Build history of the part. All positions in model axes, mm. Face numbers are marked on the shaded views. A direction names the side the tool comes from. Coordinates: 2 decimals unless noted, no trailing zeros. Order: outer loops, then holes, each group sorted by start corner. A loop starts at its lowest first (then second) coordinate and runs counter-clockwise, first axis right, second up. Notation, with made-up numbers: (19.25, 21.25) -> (68.25, 21.25) arc R33 ccw to (68.25, 54.25) -> close; hole circle Ø10 at (24.25, 24). An arc over 180 degrees is marked (long way). Write each question's results on one line, items separated by ' | '.
from build123d import *

# Parameters (mm, degrees)
F0_W     = 25
F0_H     = 1
F0_W_2   = 76
F0_W_3   = 75
F3_R     = 55
F4_DEPTH = 176
F5_R     = 75
F6_DEPTH = 1200


# Not quite as in the source:
# - a feature names something its author has since deleted; it is built from what else it names


with BuildPart() as f1:
    # F0 (on Front) → F1 (revolve)
    with BuildSketch(Plane.XZ):
        Polygon((-100, -55), (-75, -55), (-75, 126), (-76, 126), (-76, 166), (-99, 166), (-99, 126), (-100, 126), align=None)
        with Locations((-87.5, -55.5)):
            Rectangle(F0_W, F0_H)
        Polygon((-76, -164), (-75, -164), (-75, -56), (-100, -56), (-100, -164), (-99, -164), (-99, -124), (-76, -124), align=None)
    revolve(axis=Axis((0, 0, -35.4669196472), (0, 0, -1)))

    # F0 (on Front) → F2 (revolve)
    with BuildSketch(Plane.XZ):
        with Locations((-138, -55.5)):
            Rectangle(F0_W_2, F0_H)
        with Locations((-87.5, -55.5)):
            Rectangle(F0_W, F0_H)
        with Locations((-37.5, -55.5)):
            Rectangle(F0_W_3, F0_H)
    revolve(axis=Axis((-175, 0, 0), (-1, 0, 0)))

    # F3 (on face) → F4 (cut, through all)
    with BuildSketch(Plane(origin=(-176, 0, 0), x_dir=(0, -1, 0), z_dir=(-1, 0, 0))):
        Circle(F3_R)
    extrude(amount=-F4_DEPTH, mode=Mode.SUBTRACT)

    # F5 (on face) → F6 (cut)
    with BuildSketch(Plane.XY.offset(166)):
        Circle(F5_R)
    extrude(amount=-F6_DEPTH, mode=Mode.SUBTRACT)


solid = f1.part
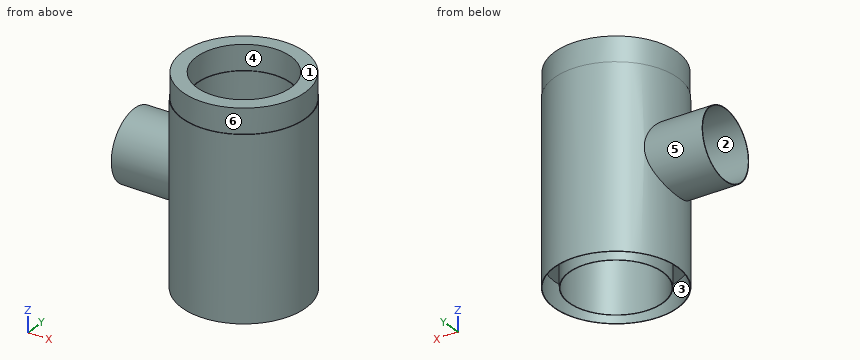
Item 1: Slice it at B-B, the plane x = 0. List the corners of the cut face in (y, z).
Answer:
outline: (-100, -164) -> (-99, -164) -> (-99, -124) -> (-76, -124) -> (-76, -164) -> (-75, -164) -> (-75, 126) -> (-76, 126) -> (-76, 166) -> (-99, 166) -> (-99, 126) -> (-100, 126) -> close; (75, -164) -> (76, -164) -> (76, -124) -> (99, -124) -> (99, -164) -> (100, -164) -> (100, 126) -> (99, 126) -> (99, 166) -> (76, 166) -> (76, 126) -> (75, 126) -> close
Item 2: Tool access for the marked faces 1 and 2: list every direction of +Z, -Z, +X, -X, +Y, -Y with a clear straight run to the whole face (end or side of a thin tool).
Answer:
face 1: +Z, +X, -X, +Y, -Y | face 2: -X
Item 3: Slice it at D-D, the plane y = -67. List the corners of the cut face in (x, z), and give its area (3 significant figures).
Answer:
outline: (-74.24, -164) -> (-72.88, -164) -> (-72.88, -124) -> (-35.87, -124) -> (-35.87, -164) -> (-33.7, -164) -> (-33.7, 126) -> (-35.87, 126) -> (-35.87, 166) -> (-72.88, 166) -> (-72.88, 126) -> (-74.24, 126) -> close; (33.7, -164) -> (35.87, -164) -> (35.87, -124) -> (72.88, -124) -> (72.88, -164) -> (74.24, -164) -> (74.24, 126) -> (72.88, 126) -> (72.88, 166) -> (35.87, 166) -> (35.87, 126) -> (33.7, 126) -> close | area: 23,500 mm^2
Item 4: Pull direction X, two halves, no side cores. Call the marked faces 3, 4, 5 and 6: released by +X, released by -X, zero draft, split by the parting line, or undercut.
Answer:
face 3: undercut | face 4: undercut | face 5: zero draft | face 6: split by the parting line
Item 5: Drill centre lines: line 1 (Y direction, x = -100, z = 0); line 2 (Y direction, x = 0, z = 141). Where is each one in solid material? Low to high. Write a range as from..to.
Answer:
line 1: y = -56..-55, 55..56 | line 2: y = -99..-76, 76..99
Item 6: Slice it at A-A, the plane y = 0. State how many separate pieces and enclosed holes the cut face has, and give its area (3 significant figures).
Answer:
separate pieces: 3 | enclosed holes: 0 | area: 11,900 mm^2
Item 7: Slice it at C-C, the plane z = -141.5. List the corners of the cut face in (x, y).
Answer:
outline: circle Ø200 at (0, 0); circle Ø152 at (0, 0); hole circle Ø198 at (0, 0); hole circle Ø150 at (0, 0)
Item 8: Pin check, flat tips, straight feed: pin 1 (5 mm diameter, centred on y = 79.5, z = 125.5, fed in from +X); pin 2 (4 mm diameter, centred on y = -79.5, z = 81.5, fed in from -X); pin 3 (6 mm diameter, centred on x = -66.5, z = -126.5, fed in from -Y). Stop position of each tip, or through.
Answer:
pin 1: stops at x = 63.8 | pin 2: stops at x = -63.2 | pin 3: stops at y = -77.25
